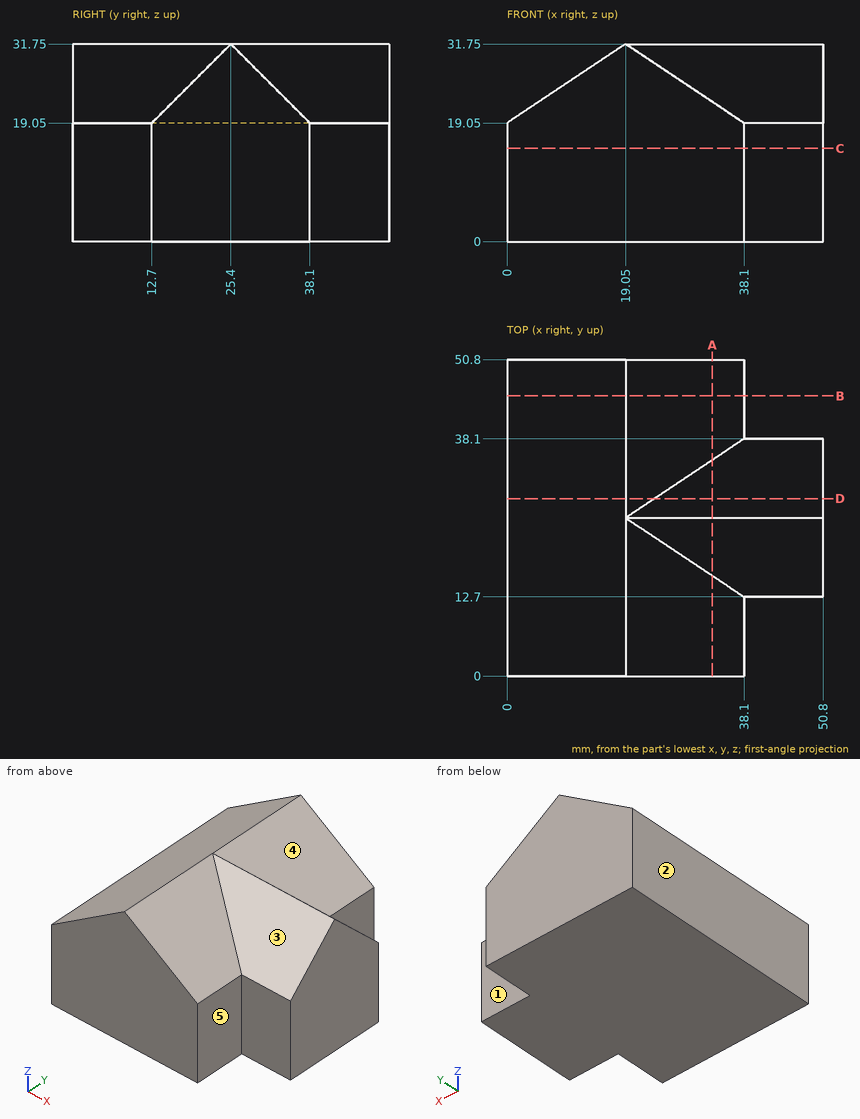
Geometry: see drawing. Coordinates: mm, zero at the bounding-box minimum. A direction names the side the tool comes from. Give positions to 0.01 mm unless a question says otherwise; leave off trailing zeros. Order: outer loops, then holes, each group sorted by start corner. A loop starts at its lowest first (then second) coordinate and runs counter-clockwise, first axis right, second up. Notation, with made-up numbers: M -3.5,61 L 2.5,61 A37 cw 2.5,100 Z; hole C -8,54.5 d10. An arc over 180 degrees is marked long. Answer as CSV lines item,"result". Start each with the question number.
1) Cut plane C-C (z = 15). Output: boundary loops of the cut face in (x, y).
2) Cut plane A-A (x = 33). Output: boundary loops of the cut face in (y, z), then the cut area to 3 significant figures.
3) Line query: line 1 (X direction, y = 6, z = 12); line 2 (Z direction, x = 45, y = 17.5); line 3 (Y direction, x = 46.5, z = 11.5). Output: solid intervals per line, ascending. Write a range as from..to.
4) First-contact query: P1, Ø10, axis at y = 6.5, z = 6.5, coming from the +X side; P2, Ø5, axis at x = 39, y = 41.5, coming from the +Z side; P3, Ø6.5, axis at x = 45.5, z = 10, coming from the +Y side. Flat tips, straight axial feed; report the tip coordinate or a pass-through.
5) Set-up query: the marked faces 1, 2, 3, 4 and 5. Return all of +Z, -Z, +X, -X, +Y, -Y with unobstructed straight access to the full face (end or side cutting, diameter ignored); none if empty.
6) Cut plane D-D (y = 28.5). Output: boundary loops of the cut face in (x, z).
7) Cut plane B-B (y = 45). Output: boundary loops of the cut face in (x, z).
Findings below:
1,outline,"M 0,0 L 38.1,0 L 38.1,12.7 L 50.8,12.7 L 50.8,38.1 L 38.1,38.1 L 38.1,50.8 L 0,50.8 Z"
2,outline,"M 0,0 L 50.8,0 L 50.8,22.45 L 34.7,22.45 L 25.4,31.75 L 16.1,22.45 L 0,22.45 Z"
2,area,"1,230 mm²"
3,line 1,"x = 0..38.1"
3,line 2,"z = 0..23.85"
3,line 3,"y = 12.7..38.1"
4,P1,"stops at x = 38.1"
4,P2,"stops at z = 20.12"
4,P3,"stops at y = 38.1"
5,face 1,"+Z, -Z, +X, +Y"
5,face 2,"+Z, -Z, -X, +Y, -Y"
5,face 3,"+Z, +X, -Y"
5,face 4,"+Z, +X, +Y"
5,face 5,"+Z, -Z, +X, -Y"
6,outline,"M 0,0 L 50.8,0 L 50.8,28.65 L 23.7,28.65 L 19.05,31.75 L 0,19.05 Z"
7,outline,"M 0,0 L 38.1,0 L 38.1,19.05 L 19.05,31.75 L 0,19.05 Z"
